The model under review builds one solid part; all positions refer to its coordinate system, in mm. A direction names the side the tool comes from. Coordinates: 2 decimals unless noted, no trailing zeros. Order: outer loops, then holes, each group sorted by start corner. A loop starts at its lowest first (then second) coordinate and runs counter-clockwise, first axis right, second up. Notation, with made-up numbers: M -19,60.5 L 15,60.5 A25 cw 15,75.5 Z; hole C 71.25,50.5 d10. An arc over 180 degrees is marked long. Answer in a Markdown table with one row per item.
from build123d import *

# Parameters (mm, degrees)
ESBO_O1_W                                            = 42
ESBO_O1_H                                            = 42
RESSALTO_EXTRUS_O1_DEPTH                             = 9
RESSALTO_EXTRUS_O2_DEPTH                             = 22
ESBO_O3_W                                            = 42
ESBO_O3_H                                            = 42
RESSALTO_EXTRUS_O3_DEPTH                             = 8
ESBO_O4_R                                            = 11
ESBO_O4_R_2                                          = 7.8
RESSALTO_EXTRUS_O4_DEPTH                             = 2
BROCA_DE_ROSQUEAR_PARA_TARRAXA_DE_M41_D              = 3.3
BROCA_DE_ROSQUEAR_PARA_TARRAXA_DE_M41_DEPTH          = 20
BROCA_DE_ROSQUEAR_PARA_TARRAXA_DE_M41_TIP            = 0.991420021
CHANFRO1_SIZE                                        = 5
REBAIXO_PARA_PARAFUSO_ALLEN_SEXTAVADO_DE_D           = 3.4
REBAIXO_PARA_PARAFUSO_ALLEN_SEXTAVADO_DE_DEPTH       = 10
REBAIXO_PARA_PARAFUSO_ALLEN_SEXTAVADO_DE_CBORE_D     = 6.5
REBAIXO_PARA_PARAFUSO_ALLEN_SEXTAVADO_DE_CBORE_DEPTH = 3.4
REBAIXO_PARA_PARAFUSO_ALLEN_SEXTAVADO_DE_TIP         = 1.021463052
ESBO_O10_R                                           = 4
BOSS_EXTRUDE1_DEPTH                                  = 660.4


with BuildPart() as part:
    # Esboço1 → Ressalto-extrusão1 (new body)
    with BuildSketch(Plane(origin=(0, 0, 0), x_dir=(1, 0, 0), z_dir=(0, 1, 0))):
        Rectangle(ESBO_O1_W, ESBO_O1_H)
    extrude(amount=RESSALTO_EXTRUS_O1_DEPTH)

    # Esboço2 → Ressalto-extrusão2 (add)
    with BuildSketch(Plane(origin=(0, 9, 0), x_dir=(1, 0, 0), z_dir=(0, 1, 0))):
        Polygon((14, 21.05), (21.05, 14), (21.05, -14), (14, -21.05), (-14, -21.05), (-21.05, -14), (-21.05, 14), (-14, 21.05), align=None)
    extrude(amount=RESSALTO_EXTRUS_O2_DEPTH)

    # Esboço3 → Ressalto-extrusão3 (add)
    with BuildSketch(Plane(origin=(0, 31, 0), x_dir=(1, 0, 0), z_dir=(0, 1, 0))):
        Rectangle(ESBO_O3_W, ESBO_O3_H)
    extrude(amount=RESSALTO_EXTRUS_O3_DEPTH)

    # Esboço4 → Ressalto-extrusão4 (add)
    with BuildSketch(Plane(origin=(0, 39, 0), x_dir=(1, 0, 0), z_dir=(0, 1, 0))):
        Circle(ESBO_O4_R)
        Circle(ESBO_O4_R_2, mode=Mode.SUBTRACT)
    extrude(amount=RESSALTO_EXTRUS_O4_DEPTH)

    # Broca de rosquear para tarraxa de M41
    with Locations(Plane(origin=(0, 39, 0), x_dir=(1, 0, 0), z_dir=(0, 1, 0))):
        with Locations((-15.5, -15.5), (-15.5, 15.5), (15.55, 15.5), (15.5, -15.5)):
            Hole(BROCA_DE_ROSQUEAR_PARA_TARRAXA_DE_M41_D / 2, depth=BROCA_DE_ROSQUEAR_PARA_TARRAXA_DE_M41_DEPTH)
            with Locations((0, 0, -(BROCA_DE_ROSQUEAR_PARA_TARRAXA_DE_M41_DEPTH + BROCA_DE_ROSQUEAR_PARA_TARRAXA_DE_M41_TIP / 2))):  # 118° drill point
                Cone(0, BROCA_DE_ROSQUEAR_PARA_TARRAXA_DE_M41_D / 2, BROCA_DE_ROSQUEAR_PARA_TARRAXA_DE_M41_TIP, mode=Mode.SUBTRACT)

    # Chanfro1
    chanfro1_edges = [part.edges().sort_by_distance(p)[0] for p in [
        (-21, 35, -21),
        (-21, 35, 21),
        (21, 35, 21),
        (21, 35, -21),
        (21, 4.5, -21),
        (-21, 4.5, -21),
        (-21, 4.5, 21),
        (21, 4.5, 21),
    ]]
    chamfer(chanfro1_edges, length=CHANFRO1_SIZE)

    # Rebaixo para parafuso Allen sextavado de M31
    with Locations(Plane(origin=(0, 0, 0), x_dir=(-1, 0, 0), z_dir=(0, -1, 0))):
        with Locations((-15.5, 15.5), (15.5, 15.5), (15.5, -15.5), (-15.5, -15.5)):
            CounterBoreHole(REBAIXO_PARA_PARAFUSO_ALLEN_SEXTAVADO_DE_D / 2, REBAIXO_PARA_PARAFUSO_ALLEN_SEXTAVADO_DE_CBORE_D / 2, REBAIXO_PARA_PARAFUSO_ALLEN_SEXTAVADO_DE_CBORE_DEPTH, depth=REBAIXO_PARA_PARAFUSO_ALLEN_SEXTAVADO_DE_DEPTH)
            with Locations((0, 0, -(REBAIXO_PARA_PARAFUSO_ALLEN_SEXTAVADO_DE_DEPTH + REBAIXO_PARA_PARAFUSO_ALLEN_SEXTAVADO_DE_TIP / 2))):  # 118° drill point
                Cone(0, REBAIXO_PARA_PARAFUSO_ALLEN_SEXTAVADO_DE_D / 2, REBAIXO_PARA_PARAFUSO_ALLEN_SEXTAVADO_DE_TIP, mode=Mode.SUBTRACT)

    # Esboço10 → Boss-Extrude1 (add)
    with BuildSketch(Plane(origin=(0, 39, 0), x_dir=(1, 0, 0), z_dir=(0, 1, 0))):
        Circle(ESBO_O10_R)
    extrude(amount=BOSS_EXTRUDE1_DEPTH)


solid = part.part
(1) Take a section at A-A (y = 641.5). Write out the cut boundary in (x, z), then the cut area to 3 significant figures.
Report:
| item | result |
|---|---|
| outline | C 0,0 d8 |
| area | 50.3 mm^2 |
(2) Insertion check: P1, Ø8, axis at x = 1.5, y = 558, coming from the +Z side; P2, Ø3, axis at y = 240, z = -5, coming from the +X side; P3, Ø2, axis at x = 17, z = -17.5, coming from the +Y side. Each pin has a flat end and moves straight along its axis. Give the tip position at first contact, or say it passes through.
Report:
| item | result |
|---|---|
| P1 | z = 4 |
| P2 | x = 1.94 |
| P3 | y = 39 |
(3) Machinability: for faces 1 (the flat face through (9, 39, 9)), 2 (the flat face through (21.05, 20, 0)), which of the approach directions +Z, -Z, +X, -X, +Y, -Y give a long, thin tool a straight path to every point of the face, cutting with its end or side? Answer none if there is none.
Report:
| item | result |
|---|---|
| face 1 | +Y |
| face 2 | +Z, -Z, +X, +Y, -Y |
(4) The part is to be moulded in two halves that separate along X. For faces 3 (the cylindrical face through (-2.38, 39.99, 10.74)), 4 (the flat face through (0, 20, 21.05)), 5 (the cylindrical face through (-5.75, 39.99, -5.27)), say which applies: +X half, -X half, draft (parallel to the pull), parting line (faces both ways), or undercut.
Report:
| item | result |
|---|---|
| face 3 | parting line |
| face 4 | draft |
| face 5 | undercut |
(5) To check wall thickness, follow line 1 (X direction, y = 2.15, z = 15.5); line 2 (Z direction, x = 15, y = 1); line 3 (Z direction, x = 15, y = 6). State the ranges of each line that lie inside material, in increasing order. Write a range as [from, to].
Report:
| item | result |
|---|---|
| line 1 | [-21, -18.75], [-12.25, 12.25], [18.75, 21] |
| line 2 | [-21, -18.71], [-12.29, 12.29], [18.71, 21] |
| line 3 | [-21, -17.12], [-13.88, 13.88], [17.12, 21] |
